Build history of the part. All positions in model axes, mm. A direction names the side the tool comes from. Give positions to 0.01 mm unless a question says otherwise; leave off trailing zeros. Write each loop counter-clockwise with the first axis right and the second up, starting at its lowest first coordinate (ties: lowest second). Pieces come first, ordered by that corner, then holes. Notation, with made-up numbers: (83.5, 35.5) -> (141.5, 35.5) arc R22 cw to (141.5, 57.5) -> close; hole circle Ø3 at (77, -8). An arc over 180 degrees is marked (long way). Put each result on its own line as item: value.
from build123d import *

# Parameters (mm, degrees)
SKETCH1_R             = 10
BOSS_EXTRUDE1_DEPTH   = 5
BOSS_EXTRUDE1_2_DEPTH = 5
BOSS_EXTRUDE2_DEPTH   = 2.5


with BuildPart() as part:
    # Sketch1 → Boss-Extrude1 (new, symmetric)
    with BuildSketch(Plane.XY):
        with BuildLine():
            ThreePointArc((-16.666666667, 52.472191289), (-40, 40), (-16.666666667, 27.527808711))
            ThreePointArc((-16.666666667, 27.527808711), (0, 32.583426132), (16.666666667, 27.527808711))
            ThreePointArc((16.666666667, 27.527808711), (40, 40), (16.666666667, 52.472191289))
            ThreePointArc((16.666666667, 52.472191289), (0, 47.416573868), (-16.666666667, 52.472191289))
        make_face()
        with Locations((-25, 40)):
            Circle(SKETCH1_R, mode=Mode.SUBTRACT)
        with Locations((25, 40)):
            Circle(SKETCH1_R, mode=Mode.SUBTRACT)
    extrude(amount=BOSS_EXTRUDE1_DEPTH, both=True)



with BuildPart() as body_2:
    # Sketch1 → Boss-Extrude1 2 (new, symmetric)
    with BuildSketch(Plane.XY):
        with BuildLine():
            ThreePointArc((16.666666667, -27.527808711), (40, -40), (16.666666667, -52.472191289))
            ThreePointArc((16.666666667, -52.472191289), (0, -47.416573868), (-16.666666667, -52.472191289))
            ThreePointArc((-16.666666667, -52.472191289), (-40, -40), (-16.666666667, -27.527808711))
            ThreePointArc((-16.666666667, -27.527808711), (0, -32.583426132), (16.666666667, -27.527808711))
        make_face()
        with Locations((25, -40)):
            Circle(SKETCH1_R, mode=Mode.SUBTRACT)
        with Locations((-25, -40)):
            Circle(SKETCH1_R, mode=Mode.SUBTRACT)
    extrude(amount=BOSS_EXTRUDE1_2_DEPTH, both=True)


with BuildPart() as part_1:
    add(part.part)

    add(body_2.part)  # Boss-Extrude2 merges body 2
    # Sketch1_3 → Boss-Extrude2 (add, symmetric)
    with BuildSketch(Plane.XY):
        with BuildLine():
            ThreePointArc((31.871842709, 26.666666667), (24.151837211, 25.023998535), (16.666666667, 27.527808711))
            ThreePointArc((16.666666667, 27.527808711), (0, 32.583426132), (-16.666666667, 27.527808711))
            ThreePointArc((-16.666666667, 27.527808711), (-24.151837211, 25.023998535), (-31.871842709, 26.666666667))
            ThreePointArc((-31.871842709, 26.666666667), (-15.615528128, 0), (-31.871842709, -26.666666667))
            ThreePointArc((-31.871842709, -26.666666667), (-24.151837211, -25.023998535), (-16.666666667, -27.527808711))
            ThreePointArc((-16.666666667, -27.527808711), (0, -32.583426132), (16.666666667, -27.527808711))
            ThreePointArc((16.666666667, -27.527808711), (24.151837211, -25.023998535), (31.871842709, -26.666666667))
            ThreePointArc((31.871842709, -26.666666667), (15.615528128, 0), (31.871842709, 26.666666667))
        make_face()
    extrude(amount=BOSS_EXTRUDE2_DEPTH, both=True)


solid = part_1.part
1) Slice it at B-B (z = 0). Write the cut outline in (x, y), plus the area to 3 significant figures.
Filled sheet:
outline: (-31.87, -26.67) arc R15 ccw (long way) to (-16.67, -52.47) arc R30 cw to (16.67, -52.47) arc R15 ccw (long way) to (31.87, -26.67) arc R30 cw to (31.87, 26.67) arc R15 ccw (long way) to (16.67, 52.47) arc R30 cw to (-16.67, 52.47) arc R15 ccw (long way) to (-31.87, 26.67) arc R30 cw to start; hole circle Ø20 at (-25, -40); hole circle Ø20 at (-25, 40); hole circle Ø20 at (25, -40); hole circle Ø20 at (25, 40)
area: 4,700 mm2
2) Slice it at D-D (x = 0). Write the cut outline in (y, z), plus the area to 3 significant figures.
Filled sheet:
outline: (-47.42, -5) -> (-32.58, -5) -> (-32.58, -2.5) -> (32.58, -2.5) -> (32.58, -5) -> (47.42, -5) -> (47.42, 5) -> (32.58, 5) -> (32.58, 2.5) -> (-32.58, 2.5) -> (-32.58, 5) -> (-47.42, 5) -> close
area: 622 mm2
3) Pin check, flat tips, straight feed: pin 1 (19 mm diameter, centred on x = 2.5, y = -1, fed in from -Z); pin 2 (23 mm diameter, centred on x = 25, y = 40, fed in from -Z); pin 3 (1.5 mm diameter, centred on x = -2.5, z = -0.5, fed in from +Y); pin 4 (6 mm diameter, centred on x = 13, z = -2.5, fed in from -Y). Stop position of each tip, or through.
Filled sheet:
pin 1: z = -2.5
pin 2: z = -5
pin 3: y = 47.59
pin 4: y = -52.04
4) Slice it at C-C (x = 20). Write the cut outline in (y, z).
Filled sheet:
outline: (-54.14, -5) -> (-48.66, -5) -> (-48.66, 5) -> (-54.14, 5) -> close; (-31.34, -5) -> (-25.86, -5) -> (-25.86, -2.5) -> (-15.62, -2.5) -> (-15.62, 2.5) -> (-25.86, 2.5) -> (-25.86, 5) -> (-31.34, 5) -> close; (15.62, -2.5) -> (25.86, -2.5) -> (25.86, -5) -> (31.34, -5) -> (31.34, 5) -> (25.86, 5) -> (25.86, 2.5) -> (15.62, 2.5) -> close; (48.66, -5) -> (54.14, -5) -> (54.14, 5) -> (48.66, 5) -> close
5) Wall check: L1, parallel to Y at x = -25, z = 2.75; L2, parallel to Y at x = -32, z = 2.25; L3, parallel to X at y = 42, z = -1.75. Give the ranges that are in metal, low to high.
Filled sheet:
L1: -55 to -50, -30 to -25, 25 to 30, 50 to 55
L2: -53.27 to -47.14, -32.86 to -26.73, 26.73 to 32.86, 47.14 to 53.27
L3: -39.87 to -34.8, -15.2 to 15.2, 34.8 to 39.87
6) Pull direction Y, two halves, no side cores. Call faces 1 (the cylindrical face through (29.614, 31.128, -0.07)), 2 (the cylindrical face through (0.247, -47.418, 0.07)), 3 (the flat face through (1, -40, 5)): released by +Y, released by -Y, zero draft, split by the parting line, or undercut.
Filled sheet:
face 1: undercut
face 2: released by -Y
face 3: zero draft
7) Slice it at A-A (y = -40). Write the cut outline in (x, z).
Filled sheet:
outline: (-40, -5) -> (-35, -5) -> (-35, 5) -> (-40, 5) -> close; (-15, -5) -> (15, -5) -> (15, 5) -> (-15, 5) -> close; (35, -5) -> (40, -5) -> (40, 5) -> (35, 5) -> close
8) Tool access for faces 4 (the cylindrical face through (-0.247, 32.582, -3.732)), 5 (the cylindrical face through (29.614, -48.872, -0.07)), 6 (the cylindrical face through (-0.247, 32.582, 3.768)): list every direction of +Z, -Z, +X, -X, +Y, -Y with a clear straight run to the whole face (end or side of a thin tool).
Filled sheet:
face 4: -Z
face 5: +Z, -Z
face 6: +Z
